Here's how the part is built. I have some questions about the finished solid (model axes, mm). A direction names the side the tool comes from. Round coordinates to 2 decimals unless told otherwise and drop trailing zeros. Loops run counter-clockwise (first coordinate to the right, second up) from the corner with the lowest first, then second, coordinate; pieces in that order, holes last. Notation, with made-up numbers: M -10,46 L 4,46 A27 ccw 4,68 Z; hole C 69.5,-29 d5. An arc over 180 degrees is marked long. Use a Markdown table: item, result.
```python
from build123d import *

# Parameters (mm, degrees)
F0_W     = 10
F0_H     = 8
F0_H_2   = 7
F1_DEPTH = 10
F2_R     = 1.8
F3_DEPTH = 10
F4_R     = 5


with BuildPart() as f1:
    # F0 (on Top) → F1 (new body)
    with BuildSketch(Plane.XY):
        Polygon((15, 36.5), (15, 37.5), (-15, 37.5), (-15, 35.5), (-15, 28.5), (-15, 18.5), (-15, 10.5), (-15, 0.5), (-15, -7.5), (-15, -37.5), (15, -37.5), (15, -7.5), (15, 0.5), (15, 10.5), (15, 18.5), (15, 28.5), align=None)
        with Locations((20, 32.5)):
            Rectangle(F0_W, F0_H)
        with Locations((-20, 32)):
            Rectangle(F0_W, F0_H_2)
        with Locations((20, 14.5)):
            Rectangle(F0_W, F0_H)
        with Locations((-20, 14.5)):
            Rectangle(F0_W, F0_H)
        with Locations((20, -3.5)):
            Rectangle(F0_W, F0_H)
        with Locations((-20, -3.5)):
            Rectangle(F0_W, F0_H)
    extrude(amount=F1_DEPTH)

    # F2 (on face) → F3 (cut)
    with BuildSketch(Plane.XY.offset(10)):
        with Locations((-10, -29.5)):
            Circle(F2_R)
        with Locations((10, -29.5)):
            Circle(F2_R)
    extrude(amount=-F3_DEPTH, mode=Mode.SUBTRACT)

    # F4
    f4_edges = [f1.edges().sort_by_distance(p)[0] for p in [
        (15, -37.5, 5),
        (-15, -37.5, 5),
    ]]
    fillet(f4_edges, radius=F4_R)


solid = f1.part
```
Q1. For faces 5 (the flat face through (-20, 28.5, 5)), 6 (the flat face through (20, 0.5, 5)), 7 (the flat face through (15, -20, 5)), which set-ups out of +Z, -Z, +X, -X, +Y, -Y let a thin tool reach every point of the face, with its end or its side?
Return value:
| item | result |
|---|---|
| face 5 | +Z, -Z, -X |
| face 6 | +Z, -Z, +X |
| face 7 | +Z, -Z, +X, -Y |
Q2. I need wall thicknesses on line 1 (Y direction, x = 10, z = 4); line 2 (X direction, y = -26, z = 1); line 3 (Y direction, x = 9, z = 2.75). Which ranges of each line are inside material? Lowest first, please. Write a range as from..to.
Return value:
| item | result |
|---|---|
| line 1 | y = -37.5..-31.3, -27.7..37.5 |
| line 2 | x = -15..15 |
| line 3 | y = -37.5..-31, -28..37.5 |
Q3. Will these pins go through, and if not, where does the flat tip stop? P1, Ø3, axis at y = 25, z = 5, coming from the +X side; P2, Ø3, axis at x = 19.5, z = 4.5, coming from the -Y side; P3, Ø3, axis at y = 25, z = 4.5, coming from the -X side; P4, Ø6, axis at x = 10, y = -29.5, coming from the -Z side.
Return value:
| item | result |
|---|---|
| P1 | stops at x = 15 |
| P2 | stops at y = -7.5 |
| P3 | stops at x = -15 |
| P4 | stops at z = 0 |
Q4. Imagine slicing it at B-B, the plane y = -29.5. Please give me the cut outline in (x, z).
Return value:
| item | result |
|---|---|
| outline | M -15,0 L -11.8,0 L -11.8,10 L -15,10 Z; M -8.2,0 L 8.2,0 L 8.2,10 L -8.2,10 Z; M 11.8,0 L 15,0 L 15,10 L 11.8,10 Z |
Q5. We'd pull the mould along Y, two halves only. Please class faces 1 (the flat face through (20, 28.5, 5)), 2 (the flat face through (-15, -20, 5)), 3 (the flat face through (0, -37.5, 5)), 4 (the flat face through (0, 37.5, 5)): pulls with the +Y half, pulls with the -Y half, needs draft (parallel to the pull), parting line crosses it, or undercut.
Return value:
| item | result |
|---|---|
| face 1 | undercut |
| face 2 | needs draft |
| face 3 | pulls with the -Y half |
| face 4 | pulls with the +Y half |
Q6. Imagine slicing it at D-D, the plane y = 6. Please give me the cut outline in (x, z), then the cut area to 3 significant figures.
Return value:
| item | result |
|---|---|
| outline | M -15,0 L 15,0 L 15,10 L -15,10 Z |
| area | 300 mm^2 |
Q7. Imagine slicing it at C-C, the plane z = 8.5. Give the number of separate pieces and of enclosed holes in the cut face, then the cut area to 3 significant figures.
Return value:
| item | result |
|---|---|
| separate pieces | 1 |
| enclosed holes | 2 |
| area | 2,690 mm^2 |
Q8. Imagine slicing it at A-A, the plane x = 21.5. Please give me the cut outline in (y, z), then the cut area to 3 significant figures.
Return value:
| item | result |
|---|---|
| outline | M -7.5,0 L 0.5,0 L 0.5,10 L -7.5,10 Z; M 10.5,0 L 18.5,0 L 18.5,10 L 10.5,10 Z; M 28.5,0 L 36.5,0 L 36.5,10 L 28.5,10 Z |
| area | 240 mm^2 |
